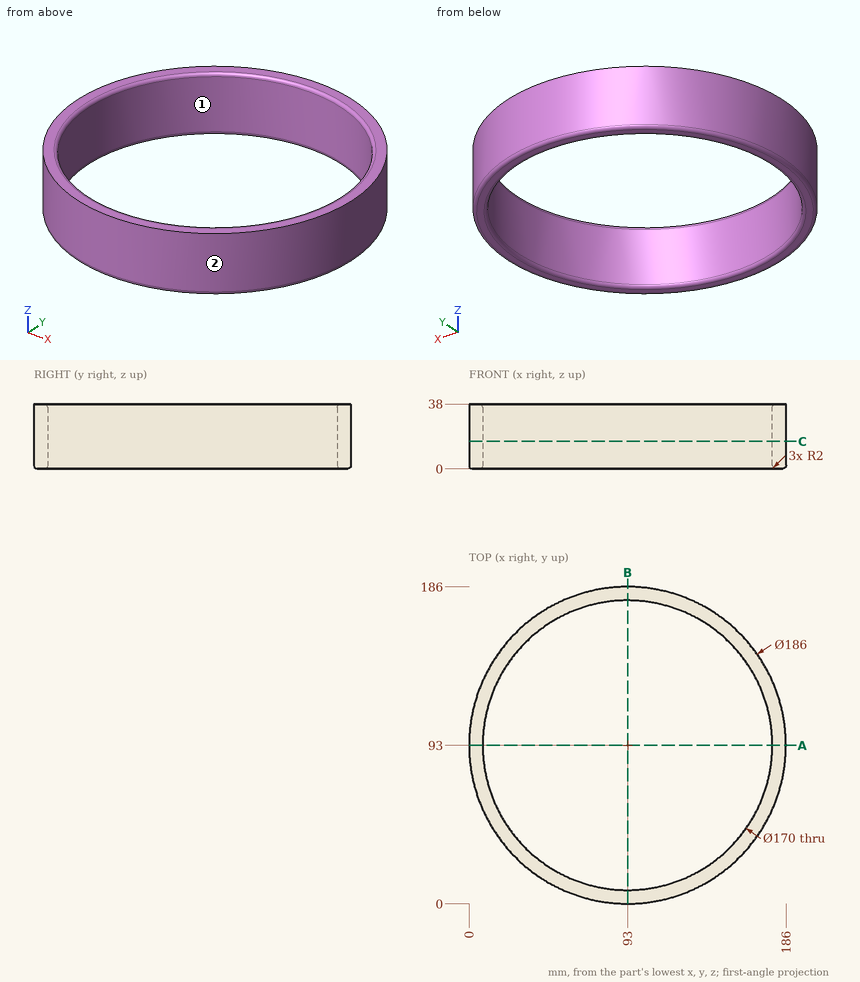
Check sheet for the drawn part. Datum: minimum x, y, z corner. Units: mm. Round coordinates to 2 decimals unless told otherwise and drop trailing zeros. Loops run counter-clockwise (first coordinate to the right, second up) from the corner with the lowest first, then second, coordinate; pieces in that order, holes last. Notation, with made-up numbers: (59.5, -5.5) -> (114.5, -5.5) arc R17 ccw to (114.5, 22.5) -> close; hole circle Ø6 at (12.5, 50). An arc over 180 degrees is marked (long way). Put each result on its own line as item: value. Start each with the question number.
1. Scan lines: probe 1 along Y at (x, z) = (93, 11); probe 2 along Y at (x, z) = (51, 19); probe 3 along X at (y, z) = (148.5, 4.5). Record each from-to range of solid material in increasing order.
2. Section check A-A (y = 93). Enter the section's corners in (x, z).
3. Section check C-C (z = 16). Enter the section's corners in (x, y).
4. Gauge pin test, flat ends, axial feed: pin 1 (3 mm diameter, centred on y = 95.5, z = 21.5, fed in from +X); pin 2 (10 mm diameter, centred on y = 22.5, z = 24, fed in from -X); pin 3 (6 mm diameter, centred on y = 158, z = 23, fed in from -X). Record the tip position at first contact, or that the pin passes through.
5. Draft check along X on the marked faces 1 and 2. Enter one of: +X half, -X half, draft (parallel to the pull), parting line (faces both ways), or undercut.
Findings:
1. probe 1: y = 0 to 8, 178 to 186
1. probe 2: y = 10.02 to 19.1, 166.9 to 175.98
1. probe 3: x = 18.38 to 28.62, 157.38 to 167.62
2. outline: (0, 2) arc R2 ccw to (2, 0) -> (6, 0) arc R2 ccw to (8, 2) -> (8, 36) arc R2 ccw to (6, 38) -> (0, 38) -> close; (178, 2) arc R2 ccw to (180, 0) -> (184, 0) arc R2 ccw to (186, 2) -> (186, 38) -> (180, 38) arc R2 ccw to (178, 36) -> close
3. outline: circle Ø186 at (93, 93); hole circle Ø170 at (93, 93)
4. pin 1: stops at x = 185.99
4. pin 2: stops at x = 26.98
4. pin 3: stops at x = 23.68
5. face 1: undercut
5. face 2: parting line
